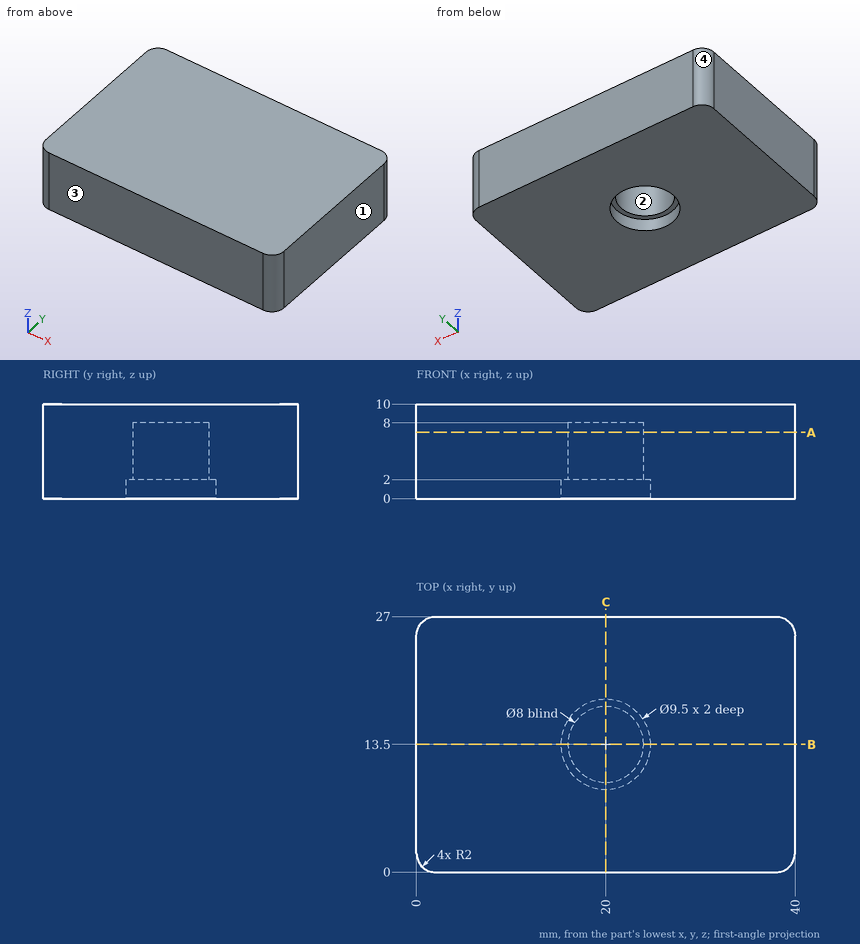
Print and shaded views of the part. All mm, measured from the part's lowest x, y and z. Give positions to 0.01 mm unless a question says otherwise; leave off trailing zeros. Loops run counter-clockwise (first coordinate to the right, second up) from the corner with the lowest first, then second, coordinate; pieces in that order, holes last. Notation, with made-up numbers: (12, 73.25) -> (36, 73.25) arc R28 cw to (36, 98.25) -> close; hole circle Ø7 at (5.25, 60.5). An arc over 180 degrees is marked (long way). Use CSV: the item, a comma, the result in double quotes. Start each with the question number.
1) Flat gauge pins, fed straight in: pin 1 Ø3 at (x, z) = (14.5, 5) entering from -Y; pin 2 Ø2.5 at (x, y) = (20.5, 14.5) entering from -Z. Where does each tip first touch, or does it go through?
2) Wall check: line 1 (Y direction, x = 20, z = 6.2); line 2 (Y direction, x = 20, z = 0.6); line 3 (X direction, y = 15.25, z = 1.25). Give the ranges that are in metal, low to high.
3) Mould opens along Y. For the marked faces 1, 2, 3 and 4 say: released by +Y, released by -Y, zero draft, split by the parting line, or undercut.
4) Slice it at A-A on z = 7. Give the cut face in (x, y), plus the area to 3 significant figures.
5) Slice it at B-B on y = 13.5. Give the cut face in (x, z).
6) Slice it at C-C on x = 20. Give the cut face in (y, z).
Computed values:
1,pin 1,"stops at y = 0"
1,pin 2,"stops at z = 8"
2,line 1,"y = 0 to 9.5, 17.5 to 27"
2,line 2,"y = 0 to 8.75, 18.25 to 27"
2,line 3,"x = 0 to 15.58, 24.42 to 40"
3,face 1,"zero draft"
3,face 2,"undercut"
3,face 3,"released by -Y"
3,face 4,"released by +Y"
4,outline,"(0, 2) arc R2 ccw to (2, 0) -> (38, 0) arc R2 ccw to (40, 2) -> (40, 25) arc R2 ccw to (38, 27) -> (2, 27) arc R2 ccw to (0, 25) -> close; hole circle Ø8 at (20, 13.5)"
4,area,"1,030 mm^2"
5,outline,"(0, 0) -> (15.25, 0) -> (15.25, 2) -> (16, 2) -> (16, 8) -> (24, 8) -> (24, 2) -> (24.75, 2) -> (24.75, 0) -> (40, 0) -> (40, 10) -> (0, 10) -> close"
6,outline,"(0, 0) -> (8.75, 0) -> (8.75, 2) -> (9.5, 2) -> (9.5, 8) -> (17.5, 8) -> (17.5, 2) -> (18.25, 2) -> (18.25, 0) -> (27, 0) -> (27, 10) -> (0, 10) -> close"
